For this review, take the finished solid that the model builds, in its own axes (mm). A direction names the side the tool comes from. Give positions to 0.01 mm unless a question says otherwise; leave off trailing zeros. Write each loop counter-clockwise with the first axis right and the second up, starting at its lowest first coordinate (ties: lowest second). Pieces come first, ordered by that corner, then holes.
Q1. We need section A-A (x = -67). Write out the cut boundary in (y, z), then the cut area to 3 significant figures.
Q2. Mouldability with a two-part tool opening along X and no side actions: class faces 4 (the cylindrical face through (73, -39, 2)), 5 (the flat face through (57, -27.3, 2)), 6 (the flat face through (-1, 1, 0)) as released by +X, released by -X, zero draft, split by the parting line, or undercut.
Q3. Insertion check: P1, Ø8.5, axis at x = -67, y = -30, coming from the +Z side; P2, Ø0.8, axis at x = 0, z = 4.5, coming from the -Y side; P3, Ø0.8, axis at y = -32.5, z = 4.5, coming from the -X side. Each pin has a flat end and moves straight along its axis. Give the tip position at first contact, or say it passes through.
Q4. We need section B-B (z = 1.5). Write out the cut boundary in (x, y), then the cut area to 3 significant figures.
Q5. For line 1 (Y direction, x = -67, z = 1.6); line 2 (Z direction, x = -62, y = 21.5); line 3 (X direction, y = 29.5, z = 3.75), list the stretches that pass through material, from the lowest coordinate up.
Q6. We need section D-D (x = -41). Write out the cut boundary in (y, z).
Q7. We need section C-C (y = 30). Write out the cut boundary in (x, z).
Q8. Machinability: for faces 1 (the flat face through (47, -30, 2)), 2 (the flat face through (0, -35, 4)), 3 (the flat face through (-27, 36, 7)), which of the approach directions +Z, -Z, +X, -X, +Y, -Y give a long, thin tool a straight path to every point of the face, cutting with its end or side? Answer none if there is none.
```python
from build123d import *

# Parameters (mm, degrees)
F0_W         = 150
F0_H         = 80
F0_R         = 2.7
F1_DEPTH     = 5
F3_DEPTH     = 2
F4_R         = 5
F5_R         = 1.99999
F6_R         = 2
F7_W         = 10
F7_H         = 10
F8_DEPTH     = 1
F9_T1_DEPTH  = 70
F9_T3_DEPTH  = 140
F9_T5_DEPTH  = 70
F9_T7_DEPTH  = 70
F9_T10_ANGLE = 90
F9_T12_ANGLE = 90
F9_T14_ANGLE = 90
F9_T16_ANGLE = 90


# Not quite as in the source:
# - a fillet or chamfer that OpenCascade refuses, or shapes differently, is made with other operations: its cross-section is extruded or revolved along the edge and cut away or added
# - a fillet or chamfer is up to 0.001 mm smaller than in the source, because OpenCascade refuses the exact size
# - a feature names something its author has since deleted; it is built from what else it names


with BuildPart() as f1:
    # F0 (on Top) → F1 (new body)
    with BuildSketch(Plane.XY):
        Rectangle(F0_W, F0_H)
        with Locations((-67, -30)):
            Circle(F0_R, mode=Mode.SUBTRACT)
        with BuildLine():
            ThreePointArc((67, -27.3), (68.9091883092, -28.0908116908), (69.7, -30))
            ThreePointArc((69.7, -30), (68.9091883092, -31.9091883092), (67, -32.7))
            Line((67, -32.7), (47, -32.7))
            Line((47, -32.7), (47, -27.3))
            Line((47, -27.3), (67, -27.3))
        make_face(mode=Mode.SUBTRACT)
        with Locations((-67, 30)):
            Circle(F0_R, mode=Mode.SUBTRACT)
        with Locations((67, 30)):
            Circle(F0_R, mode=Mode.SUBTRACT)
    extrude(amount=F1_DEPTH)

    # F2 (on face) → F3 (join)
    with BuildSketch(Plane.XY.offset(5)):
        Polygon((-50.3, -35.3), (-50.3, 35.3), (40.3, 35.3), (40.3, 37.3), (-52.3, 37.3), (-52.3, -35.3), align=None)
    extrude(amount=F3_DEPTH)

    # F4
    f4_edges = [f1.edges().sort_by_distance(p)[0] for p in [
        (75, -40, 2.5),
        (-75, -40, 2.5),
        (-75, 40, 2.5),
        (75, 40, 2.5),
    ]]
    fillet(f4_edges, radius=F4_R)

    # F5 (radius 2 in the source; OpenCascade refuses exactly that, so slightly less here)
    f5_edges = [f1.edges().sort_by_distance(p)[0] for p in [
        (-51.3, -35.3, 7),
        (40.3, 36.3, 7),
    ]]
    fillet(f5_edges, radius=F5_R)

    # F6
    f6_edges = [f1.edges().sort_by_distance(p)[0] for p in [
        (-52.3, 37.3, 6),
    ]]
    fillet(f6_edges, radius=F6_R)

    # F7 (on face) → F8 (cut)
    with BuildSketch(Plane.XY.offset(5)):
        with Locations((0, -35)):
            Rectangle(F7_W, F7_H)
    extrude(amount=-F8_DEPTH, mode=Mode.SUBTRACT)

    # F9: fillet of radius 2 on 7 edges, made by hand

    # F9_s2 → F9_t1 (cut)
    with BuildSketch(Plane.XZ.offset(-35)):
        with BuildLine():
            ThreePointArc((-73, 5), (-74.4142135624, 4.4142135624), (-75, 3))
            Line((-75, 3), (-75, 5))
            Line((-75, 5), (-73, 5))
        make_face()
        with BuildLine():
            ThreePointArc((73, 5), (74.4142135624, 4.4142135624), (75, 3))
            Line((75, 3), (75, 5))
            Line((75, 5), (73, 5))
        make_face()
    extrude(amount=F9_T1_DEPTH, mode=Mode.SUBTRACT)

    # F9_s4 → F9_t3 (cut)
    with BuildSketch(Plane.YZ.offset(-70)):
        with BuildLine():
            ThreePointArc((38, 5), (39.4142135624, 4.4142135624), (40, 3))
            Line((40, 3), (40, 5))
            Line((40, 5), (38, 5))
        make_face()
    extrude(amount=F9_T3_DEPTH, mode=Mode.SUBTRACT)

    # F9_s6 → F9_t5 (cut)
    with BuildSketch(Plane.YZ):
        with BuildLine():
            ThreePointArc((-38, 5), (-39.4142135624, 4.4142135624), (-40, 3))
            Line((-40, 3), (-40, 5))
            Line((-40, 5), (-38, 5))
        make_face()
    extrude(amount=F9_T5_DEPTH, mode=Mode.SUBTRACT)

    # F9_s8 → F9_t7 (cut)
    with BuildSketch(Plane.YZ.offset(-70)):
        with BuildLine():
            ThreePointArc((-38, 5), (-39.4142135624, 4.4142135624), (-40, 3))
            Line((-40, 3), (-40, 5))
            Line((-40, 5), (-38, 5))
        make_face()
    extrude(amount=F9_T7_DEPTH, mode=Mode.SUBTRACT)

    # F9_s9 → F9_t10 (revolve, cut)
    with BuildSketch(Plane.XZ.offset(35)):
        with BuildLine():
            ThreePointArc((-73, 5), (-74.4142135624, 4.4142135624), (-75, 3))
            Line((-75, 3), (-75, 5))
            Line((-75, 5), (-73, 5))
        make_face()
    revolve(axis=Axis((-70, -35, 5), (0, 0, 1)), revolution_arc=F9_T10_ANGLE, mode=Mode.SUBTRACT)

    # F9_s11 → F9_t12 (revolve, cut)
    with BuildSketch(Plane.XZ.offset(35)):
        with BuildLine():
            ThreePointArc((73, 5), (74.4142135624, 4.4142135624), (75, 3))
            Line((75, 3), (75, 5))
            Line((75, 5), (73, 5))
        make_face()
    revolve(axis=Axis((70, -35, 5), (0, 0, -1)), revolution_arc=F9_T12_ANGLE, mode=Mode.SUBTRACT)

    # F9_s13 → F9_t14 (revolve, cut)
    with BuildSketch(Plane.YZ.offset(70)):
        with BuildLine():
            ThreePointArc((38, 5), (39.4142135624, 4.4142135624), (40, 3))
            Line((40, 3), (40, 5))
            Line((40, 5), (38, 5))
        make_face()
    revolve(axis=Axis((70, 35, 5), (0, 0, -1)), revolution_arc=F9_T14_ANGLE, mode=Mode.SUBTRACT)

    # F9_s15 → F9_t16 (revolve, cut)
    with BuildSketch(Plane.YZ.offset(-70)):
        with BuildLine():
            ThreePointArc((38, 5), (39.4142135624, 4.4142135624), (40, 3))
            Line((40, 3), (40, 5))
            Line((40, 5), (38, 5))
        make_face()
    revolve(axis=Axis((-70, 35, 5), (0, 0, 1)), revolution_arc=F9_T16_ANGLE, mode=Mode.SUBTRACT)


solid = f1.part
```
Computed:
1. outline: (-40, 0) - (-32.7, 0) - (-32.7, 5) - (-38, 5) arc R2 ccw to (-40, 3) - close; (-27.3, 0) - (27.3, 0) - (27.3, 5) - (-27.3, 5) - close; (32.7, 0) - (40, 0) - (40, 3) arc R2 ccw to (38, 5) - (32.7, 5) - close
1. area: 344 mm2
2. face 4: released by +X
2. face 5: undercut
2. face 6: zero draft
3. P1: stops at z = 5
3. P2: stops at y = -30
3. P3: stops at x = -74.67
4. outline: (-75, -35) arc R5 ccw to (-70, -40) - (70, -40) arc R5 ccw to (75, -35) - (75, 35) arc R5 ccw to (70, 40) - (-70, 40) arc R5 ccw to (-75, 35) - close; hole circle Ø5.4 at (-67, -30); hole circle Ø5.4 at (-67, 30); hole (47, -32.7) - (67, -32.7) arc R2.7 ccw to (67, -27.3) - (47, -27.3) - close; hole circle Ø5.4 at (67, 30)
4. area: 11,800 mm2
5. line 1: y = -40 to -32.7, -27.3 to 27.3, 32.7 to 40
5. line 2: z = 0 to 5
5. line 3: x = -74.85 to -69.65, -64.35 to 64.35, 69.65 to 74.85
6. outline: (-40, 0) - (40, 0) - (40, 3) arc R2 ccw to (38, 5) - (37.3, 5) - (37.3, 7) - (35.3, 7) - (35.3, 5) - (-38, 5) arc R2 ccw to (-40, 3) - close
7. outline: (-75, 0) - (-69.7, 0) - (-69.7, 5) - (-73, 5) arc R2 ccw to (-75, 3) - close; (-64.3, 0) - (64.3, 0) - (64.3, 5) - (-50.3, 5) - (-50.3, 7) - (-52.3, 7) - (-52.3, 5) - (-64.3, 5) - close; (69.7, 0) - (75, 0) - (75, 3) arc R2 ccw to (73, 5) - (69.7, 5) - close
8. face 1: +Z, -Z
8. face 2: +Z, -Y
8. face 3: +Z, +X, -X, +Y, -Y
